Autodesk Inventor part; units mm, degrees
ref_plane "YZ Plane" through (0, 0, 0) normal (1, 0, 0) x (0, 1, 0)
ref_plane "XZ Plane" through (0, 0, 0) normal (0, 1, 0) x (-1, 0, 0)
ref_plane "XY Plane" through (0, 0, 0) normal (0, 0, 1) x (1, 0, 0)
sketch "Boceto1" plane through (0, 0, 0) normal (0, 1, 0) x (-1, 0, 0)
  line L0 (0, 0) -> (1.4, 0)
  line L1 (1.4, 0) -> (1.4, -37)
  line L2 (1.4, -37) -> (0, -42.6)
  line L3 (0, -42.6) -> (0, 0)
  dimension "d0" = 1.4
  dimension "d1" = 5.6
  dimension "d2" = 42.6
revolve "Revolución1" add sketch "Boceto1" angle 360 about axis through (0, 0, -42.6) along (0, 0, 1)
sketch "Boceto2" plane through (0, 0, 0) normal (0, 1, 0) x (-1, 0, 0)
  line L0 (-1.4, 0) -> (-1.4, -37)
  line L1 (-1.4, -5.6) -> (-9, -5.6)
  line L2 (-9, -5.6) -> (-9, -6.4)
  line L3 (-9, -6.4) -> (-1.4, -6.4)
  line L4 (-1.4, -5.6) -> (-1.4, -6.4)
  line L5 (-1.4, 0) -> (1.4, 0)
  line L6 (0, 0) -> (0, -42.6)
  line L7 (1.4, -37) -> (0, -42.6)
  dimension "d4" = 0.8
  dimension "d5" = 7.6
  dimension "d6" = 5.6
coil "Bobina1" sketch "Boceto2" operation add axis through (0, 0, 0) along (0, 0, -1) pitch 8.6667 turns 3 hand right
properties part number "Pieza de practica 8"
Read the model definition and answer for the solid it produces. Units are mm, in the model's axes. A direction names the side the tool comes from. Coordinates: 2 decimals unless noted, no trailing zeros. Write each loop counter-clockwise with the first axis right and the second up, starting at its lowest first coordinate (ties: lowest second). Pieces come first, ordered by that corner, then holes. Notation, with made-up numbers: (2.5, -11.75) - (14.5, -11.75) arc R17 cw to (14.5, -4.75) - close; hole circle Ø5 at (47, 26). An arc over 180 degrees is marked (long way). One line per question, with ' | ' between items.
Q1. Each of these flat-tipped pins is pushed along its axis until it touches: P1, Ø2, axis at x = -4, z = -6, coming from the +Y side; P2, Ø1.5, axis at x = 0, y = -6, coming from the -Z side; P3, Ø0.9, axis at x = 3.5, z = -6, coming from the +Y side; P4, Ø8, axis at x = 6.5, z = -18, coming from the -Y side. Where does it stop, or does it pass through?
Result set:
P1: through | P2: z = -26.07 | P3: y = 0 | P4: y = -8.59
Q2. Consider L1, parallel to Z at x = 2, y = -5.75; L2, parallel to Z at x = 5.75, y = 6.75; L3, parallel to X at y = 0, z = -18. Determine where each line is inside the solid, lowest interval first. Write a range as [from, to].
Result set:
L1: [-25.44, -24.64], [-16.77, -15.97], [-8.1, -7.3] | L2: [-31.21, -30.41], [-22.54, -21.74], [-13.87, -13.07] | L3: [-1.4, 1.4]
Q3. Find section C-C, the plane z = -33.5. Write down the section's boundary in (x, y), plus the area to 3 significant figures.
Result set:
outline: circle Ø2.8 at (0, 0) | area: 6.16 mm^2
Q4. Find section A-A, the plane y = -6.5. State how many separate pieces and enclosed holes the cut face has, plus the area to 3 significant figures.
Result set:
separate pieces: 3 | enclosed holes: 0 | area: 29.9 mm^2
Q5. For faces 1 (the flat face through (5, 0, -6)), 2 (the flat face through (0, 0, 0)), 3 (the flat face through (5, 0, -32)), determine the directions among +Z, -Z, +X, -X, +Y, -Y from which every point of the face is accessible in a straight line to the end or side of a thin tool.
Result set:
face 1: +Z, +X, +Y | face 2: +Z, +X, -X, +Y, -Y | face 3: -Z, +X, -Y
